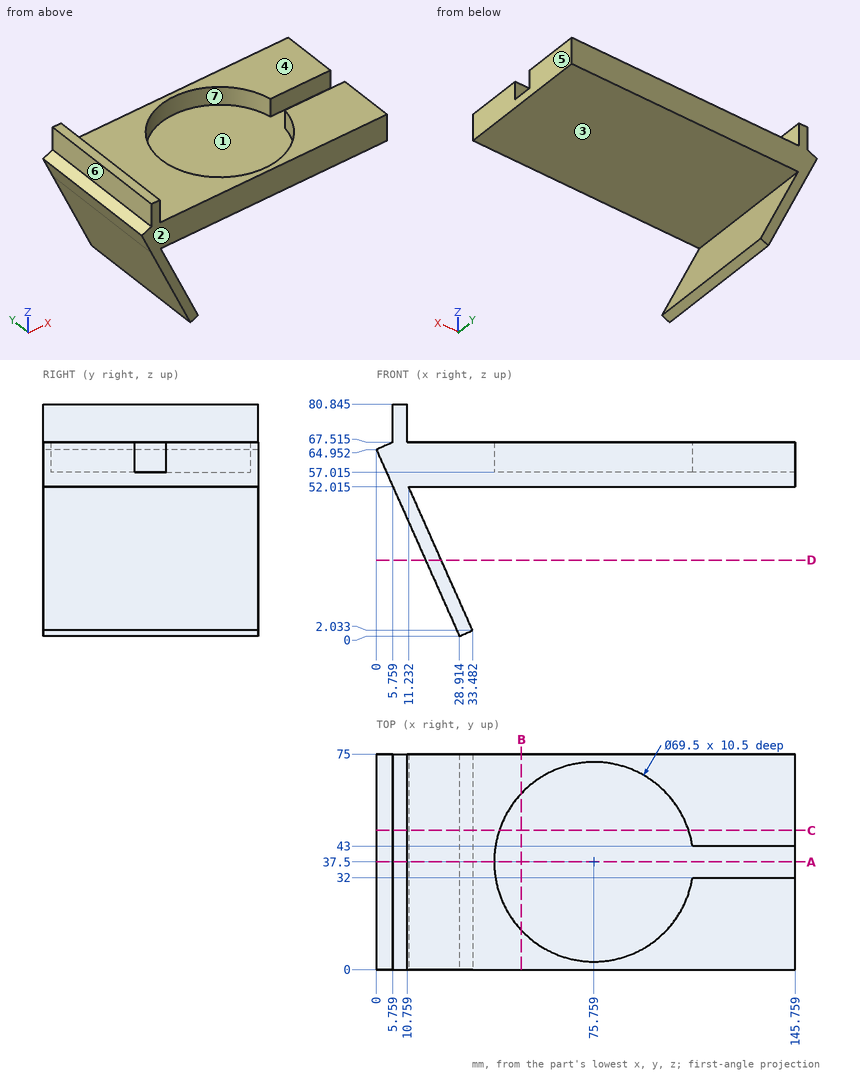
Verification items for this drawing (mm, ordinates from the low corner). A direction names the side the tool comes from. Give positions to 0.01 mm unless a question says otherwise; leave off trailing zeros. Loops run counter-clockwise (first coordinate to the right, second up) from the corner with the lowest first, then second, coordinate; pieces in that order, holes last. Notation, with made-up numbers: M -30.5,79 L 10.5,79 A29 cw 10.5,105 Z; hole C 13.5,-1 d8. An arc over 180 degrees is marked long. Answer as a JSON object with one key per item and string values. Group by question number.
Q1. Release check for a two-part mould opening along X. For the marked faces 5, 6 and 7 record: released by +X, released by -X, zero draft, split by the parting line, or undercut.
Q2. Cross-section at C-C on y = 48.5. Record the cut outline in (x, z) (1 decimal), then the cut area to 3 significant figures.
Q3. Cross-section at A-A on y = 37.5. Record the cut outline in (x, z) (1 decimal), then the cut area to 3 significant figures.
Q4. Access from +Z, -Z, +X, -X, +Y, -Y to the whole of each face (thin tool, end or side, straight path). Record for the marked faces 1, 2, 3 and 4.
Q5. Material ranges on line 1 along Z through (x, y) = (124, 56.5) (1 decimal); line 2 along Z through (x, y) = (62.5, 11.5) (1 decimal); line 3 along Z through (x, y) = (18.5, 34) (1 decimal), recorded low to high. Write a range as [from, to].
Q6. Go/stop test with flat-tipped pins: P1, Ø5, axis at x = 44.5, y = 43, coming from the -Z side (1 decimal); P2, Ø12, axis at x = 66, z = 44, coming from the +Y side; P3, Ø10, axis at y = 16, z = 34.5, coming from the +X side (1 decimal); P4, Ø3, axis at x = 122, z = 61, coming from the -Y side. Record where each tip stops, or that it passes through.
Q7. Cross-section at D-D on z = 26.5. Record the cut outline in (x, y).
Q8. Cross-section at B-B on x = 50.5. Record the cut outline in (y, z) (1 decimal).
Evaluation:
{
 "1": {"face 5": "released by +X", "face 6": "released by -X", "face 7": "undercut"},
 "2": {"outline": "M 0,65 L 28.9,0 L 33.5,2 L 11.2,52 L 145.8,52 L 145.8,67.5 L 108.7,67.5 L 108.7,57 L 42.8,57 L 42.8,67.5 L 10.8,67.5 L 10.8,80.8 L 5.8,80.8 L 5.8,67.5 Z", "area": "1,870 mm2"},
 "3": {"outline": "M 0,65 L 28.9,0 L 33.5,2 L 11.2,52 L 145.8,52 L 145.8,57 L 41,57 L 41,67.5 L 10.8,67.5 L 10.8,80.8 L 5.8,80.8 L 5.8,67.5 Z", "area": "1,460 mm2"},
 "4": {"face 1": "+Z", "face 2": "+Z, -Z, +X, -X, -Y", "face 3": "+X, +Y, -Y", "face 4": "+Z, +X, +Y, -Y"},
 "5": {"line 1": "z = [52, 67.5]", "line 2": "z = [52, 57]", "line 3": "z = [23.4, 35.7], [52, 67.5]"},
 "6": {"P1": "stops at z = 52", "P2": "passes through", "P3": "stops at x = 21.3", "P4": "stops at y = 0"},
 "7": {"outline": "M 17.12,0 L 22.59,0 L 22.59,75 L 17.12,75 Z"},
 "8": {"outline": "M 0,52 L 75,52 L 75,67.5 L 61.4,67.5 L 61.4,57 L 13.6,57 L 13.6,67.5 L 0,67.5 Z"}
}
